Design review of the part built by this model. Coordinates are the model's own, in mm. A direction names the side the tool comes from. Coordinates: 2 decimals unless noted, no trailing zeros. Order: outer loops, then holes, each group sorted by start corner. A loop starts at its lowest first (then second) coordinate and runs counter-clockwise, first axis right, second up. Notation, with made-up numbers: (36.5, 62) -> (52.5, 62) arc R23 cw to (52.5, 77) -> close; hole circle Ø1 at (-16, 29.25). An arc over 180 degrees is marked (long way). Write item = value, one per line.
```python
from build123d import *

# Parameters (mm, degrees)
F1_DEPTH = 17.5
F2_T     = -2.5


with BuildPart() as f1:
    # F0 (on Top) → F1 (new body)
    with BuildSketch(Plane.XY):
        with BuildLine():
            Line((50.0531097949, 87.5149464011), (12.6002141586, 87.5149464011))
            ThreePointArc((12.6002141586, 87.5149464011), (0.2029747702, 96.1006367998), (-12.1942646181, 87.5149464011))
            Line((-12.1942646181, 87.5149464011), (-49.7552318573, 87.5149464011))
            ThreePointArc((-49.7552318573, 87.5149464011), (-54.7049793256, 85.4646938694), (-56.7552318573, 80.5149464011))
            Line((-56.7552318573, 80.5149464011), (-56.7552318573, -91.4975939512))
            ThreePointArc((-56.7552318573, -91.4975939512), (-55.349344407, -94.8917065009), (-51.9552318573, -96.2975939512))
            Line((-51.9552318573, -96.2975939512), (52.2531097949, -96.2975939512))
            ThreePointArc((52.2531097949, -96.2975939512), (55.6472223446, -94.8917065009), (57.0531097949, -91.4975939512))
            Line((57.0531097949, -91.4975939512), (57.0531097949, 80.5149464011))
            ThreePointArc((57.0531097949, 80.5149464011), (55.0028572632, 85.4646938694), (50.0531097949, 87.5149464011))
        make_face()
    extrude(amount=F1_DEPTH)

    # F2
    f2_openings = [f1.faces().sort_by_distance(p)[0] for p in [
        (0.149336, -3.73706, 17.5),
        (0.149336, -3.73706, 0),
    ]]
    offset(amount=F2_T, openings=f2_openings, kind=Kind.INTERSECTION)


solid = f1.part
```
(1) The part is to be moulded in two halves that separate along Y. For faces 1 (the cylindrical face through (-55.39, -94.85, 8.63)), 2 (the flat face through (55, 22, 0)), 3 (the flat face through (-1, -93.798, 9)), say which applies: released by +Y, released by -Y, zero draft, split by the parting line, or undercut.
Report:
face_1 = released by -Y
face_2 = zero draft
face_3 = undercut
(2) We need section C-C (y = 9.5). Write out the cut boundary in (x, z), and give its area (3 significant figures).
Report:
outline = (-56.76, 0) -> (-54.26, 0) -> (-54.26, 17.5) -> (-56.76, 17.5) -> close; (54.55, 0) -> (57.05, 0) -> (57.05, 17.5) -> (54.55, 17.5) -> close
area = 87.5 mm²
(3) Insertion check: pin 1 (9 mm diameter, centred on x = -30, z = 12.5, fed in from +Y). The pin has a flat end and moves straight along its axis. Give the tip position at first contact, or say it passes through.
Report:
pin_1 = 87.51
(4) For faces 4 (the flat face through (32, 87.515, 9)), 5 (the flat face through (-56.755, -4, 9)), 6 (the cylindrical face through (-52.902, 83.732, 8.628)), list the 3-axis set-ups (+Z, -Z, +X, -X, +Y, -Y) from which the entire face can be reached by the end or side of a thin tool; tool diameter is ignored.
Report:
face_4 = +Z, -Z, +X, +Y
face_5 = +Z, -Z, -X, +Y, -Y
face_6 = +Z, -Z
(5) We need section B-B (x = 33). Write out the cut boundary in (y, z).
Report:
outline = (-96.3, 0) -> (-93.8, 0) -> (-93.8, 17.5) -> (-96.3, 17.5) -> close; (85.01, 0) -> (87.51, 0) -> (87.51, 17.5) -> (85.01, 17.5) -> close
(6) For L1, parallel to Y at x = -38, z = 4.75; L2, parallel to X at y = -63, z = 13.25; L3, parallel to Y at x = -8.5, z = 5.5, list the stretches that pass through material, from the lowest coordinate up.
Report:
L1 = -96.3 to -93.8, 85.01 to 87.51
L2 = -56.76 to -54.26, 54.55 to 57.05
L3 = -96.3 to -93.8, 89.16 to 92.84
(7) We need section A-A (z = 14.25). Write out the cut boundary in (x, y), and give its area (3 significant figures).
Report:
outline = (-56.76, -91.5) arc R4.8 ccw to (-51.96, -96.3) -> (52.25, -96.3) arc R4.8 ccw to (57.05, -91.5) -> (57.05, 80.51) arc R7 ccw to (50.05, 87.51) -> (12.6, 87.51) arc R13.24 ccw to (-12.19, 87.51) -> (-49.76, 87.51) arc R7 ccw to (-56.76, 80.51) -> close; hole (-54.26, -91.5) arc R2.3 ccw to (-51.96, -93.8) -> (52.25, -93.8) arc R2.3 ccw to (54.55, -91.5) -> (54.55, 80.51) arc R4.5 ccw to (50.05, 85.01) -> (10.73, 85.01) arc R10.74 ccw to (-10.32, 85.01) -> (-49.76, 85.01) arc R4.5 ccw to (-54.26, 80.51) -> close
area = 1,460 mm²
